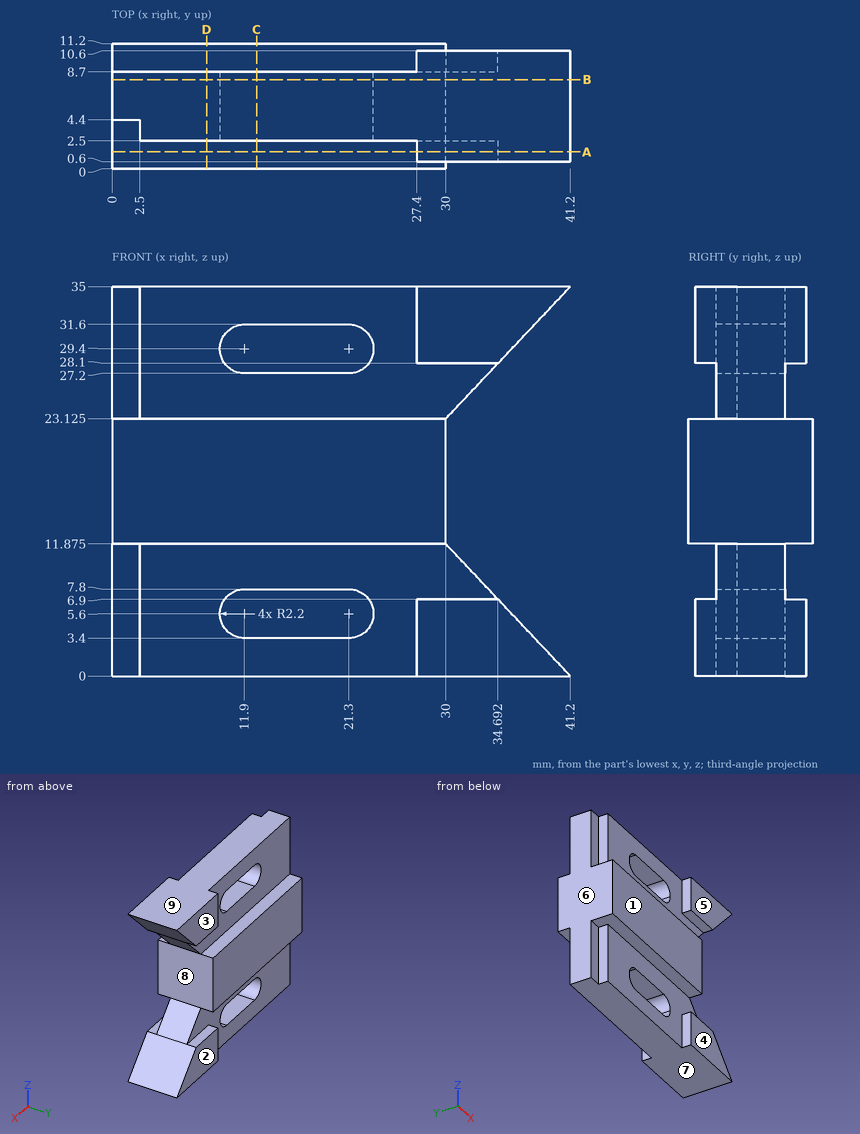
Check sheet for the drawn part. Datum: minimum x, y, z corner. Units: mm. A direction names the side the tool comes from. Coordinates: 2 decimals unless noted, no trailing zeros. Loops run counter-clockwise (first coordinate to the right, second up) from the corner with the lowest first, then second, coordinate; pieces in that order, holes last. Notation, with made-up numbers: M 20,22 L 33,22 A23 ccw 33,30 Z; hole C -23.5,18 d10. An arc over 180 degrees is marked long. Answer as a JSON object with one key per item and string values.
1. Release check for a two-part mould opening along Z. For the marked faces 6, 7, 8 and 9 record: pulls with the +Z half, pulls with the -Z half, needs draft (parallel to the pull), parting line crosses it, or undercut.
Outcome:
{"face 6": "needs draft", "face 7": "pulls with the -Z half", "face 8": "undercut", "face 9": "pulls with the +Z half"}
2. Access from +Z, -Z, +X, -X, +Y, -Y to the whole of each face (thin tool, end or side, straight path). Record for the marked faces 1, 2, 3, 4 and 5.
Outcome:
{"face 1": "+Z, -Z, +X, -X, -Y", "face 2": "-Z, +X, -X, +Y", "face 3": "+Z, +X, -X, +Y", "face 4": "-Z, +X, -X, -Y", "face 5": "+Z, +X, -X, -Y"}
3. Sectioned sample at B-B on y = 8. Record the cut outline in (x, z) (1 decimal), and give its area (3 significant figures).
Outcome:
{"outline": "M 0,0 L 41.2,0 L 30,11.9 L 30,23.1 L 41.2,35 L 0,35 Z; hole M 11.9,3.4 L 21.3,3.4 A2.2 ccw 21.3,7.8 L 11.9,7.8 A2.2 ccw Z; hole M 11.9,27.2 L 21.3,27.2 A2.2 ccw 21.3,31.6 L 11.9,31.6 A2.2 ccw Z", "area": "1,070 mm²"}
4. Scan lines: L1, parallel to Z at x = 16.5, y = 8; L2, parallel to Z at x = 22, y = 5 (1 decimal); L3, parallel to Z at x = 34.5, y = 10.5. Record each from-to range of solid material in increasing order. Write a range as from..to.
Outcome:
{"L1": "0..3.4, 7.8..27.2, 31.6..35", "L2": "0..3.5, 7.7..27.3, 31.5..35", "L3": "0..6.9, 28.1..35"}
5. Depth check by flat-ended pin: P1, Ø9.5, axis at x = 16.5, z = 31.5, coming from the -Y side; P2, Ø12, axis at x = 14, z = 31, coming from the +Y side; P3, Ø0.8, axis at x = 1, z = 7, coming from the -Y side. Enter the tip coordinate at first touch or a pass-through.
Outcome:
{"P1": "y = 2.5", "P2": "y = 8.7", "P3": "y = 4.4"}
6. Sectioned sample at A-A on y = 1.5. Record the cut outline in (x, z) (1 decimal).
Outcome:
{"outline": "M 0,11.9 L 30,11.9 L 30,23.1 L 0,23.1 Z; M 27.4,0 L 41.2,0 L 34.7,6.9 L 27.4,6.9 Z; M 27.4,28.1 L 34.7,28.1 L 41.2,35 L 27.4,35 Z"}
7. Sectioned sample at D-D on x = 8.5. Record the cut outline in (y, z) (3 decimals), and give its area (3 significant figures).
Outcome:
{"outline": "M 0,11.875 L 2.5,11.875 L 2.5,0 L 8.7,0 L 8.7,11.875 L 11.2,11.875 L 11.2,23.125 L 8.7,23.125 L 8.7,35 L 2.5,35 L 2.5,23.125 L 0,23.125 Z", "area": "273 mm²"}
8. Sectioned sample at C-C on x = 13. Record the cut outline in (y, z) (3 decimals).
Outcome:
{"outline": "M 0,11.875 L 2.5,11.875 L 2.5,7.8 L 8.7,7.8 L 8.7,11.875 L 11.2,11.875 L 11.2,23.125 L 8.7,23.125 L 8.7,27.2 L 2.5,27.2 L 2.5,23.125 L 0,23.125 Z; M 2.5,0 L 8.7,0 L 8.7,3.4 L 2.5,3.4 Z; M 2.5,31.6 L 8.7,31.6 L 8.7,35 L 2.5,35 Z"}
